Input: dimensioned drawing with shaded views. Units: mm. Origin: part minimum x, y, z. Give positions to 0.01 mm unless a question says otherwise; leave off trailing zeros. Loops run counter-clockwise (first coordinate to the right, second up) from the corner with the lowest first, then second, coordinate; pieces in that order, holes last. Notation, with made-up numbers: (61, 79.25) -> (83, 79.25) arc R14 ccw to (83, 93.25) -> close; hole circle Ø9 at (10, 66). An arc over 180 degrees is marked (long way). Answer as a JSON object with one key per item and string values.
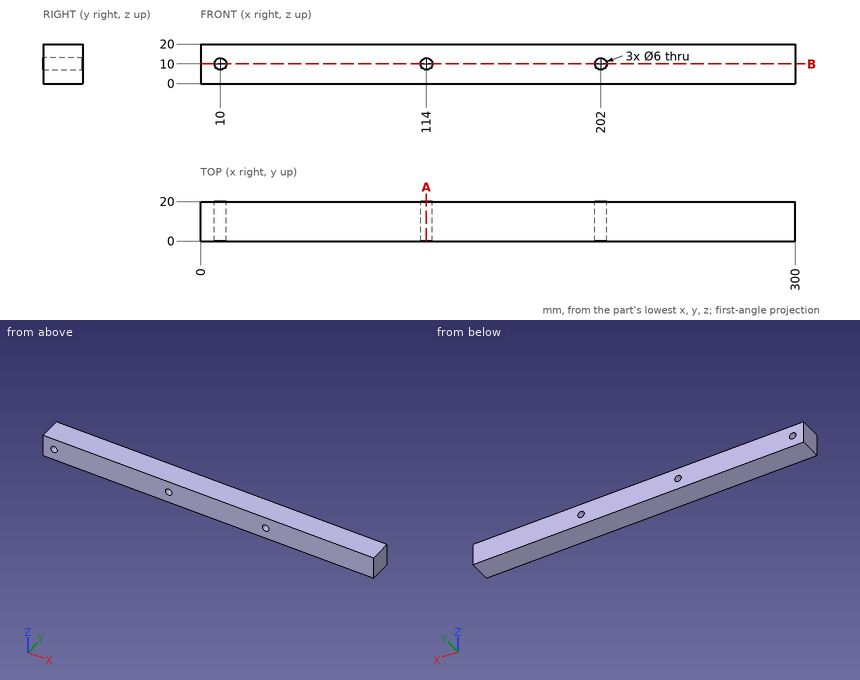
Q1. Section A-A, the plane x = 114. Return the cut outline in (y, z), then the cut area to 3 significant figures.
Evaluation:
{"outline": "(0, 0) -> (20, 0) -> (20, 7) -> (0, 7) -> close; (0, 13) -> (20, 13) -> (20, 20) -> (0, 20) -> close", "area": "280 mm2"}
Q2. Ray query, line 1 along X through (y, z) = (8, 10); line 2 along X through (y, z) = (7.5, 7.5); line 3 along Z through (x, y) = (202, 10.75). Return the intervals inside material, ascending.
Evaluation:
{"line 1": "x = 0 to 7, 13 to 111, 117 to 199, 205 to 300", "line 2": "x = 0 to 8.34, 11.66 to 112.34, 115.66 to 200.34, 203.66 to 300", "line 3": "z = 0 to 7, 13 to 20"}
Q3. Section B-B, the plane z = 10. Return the cut outline in (x, y), then the cut area to 3 significant figures.
Evaluation:
{"outline": "(0, 0) -> (7, 0) -> (7, 20) -> (0, 20) -> close; (13, 0) -> (111, 0) -> (111, 20) -> (13, 20) -> close; (117, 0) -> (199, 0) -> (199, 20) -> (117, 20) -> close; (205, 0) -> (300, 0) -> (300, 20) -> (205, 20) -> close", "area": "5,640 mm2"}
